Here's how the part is built. I have some questions about the finished solid (model axes, mm). Give positions to 0.01 mm unless a question says otherwise; leave off trailing zeros. Write each loop counter-clockwise with the first axis right and the second up, starting at its lowest first coordinate (ties: lowest second). Pieces come first, ordered by that corner, then holes. Notation, with made-up numbers: (73, 44) - (92, 44) arc R15 ccw to (92, 71) - close; hole circle Ø2 at (77.5, 58). An arc over 180 degrees is marked (long way). Use a Markdown table: item, result.
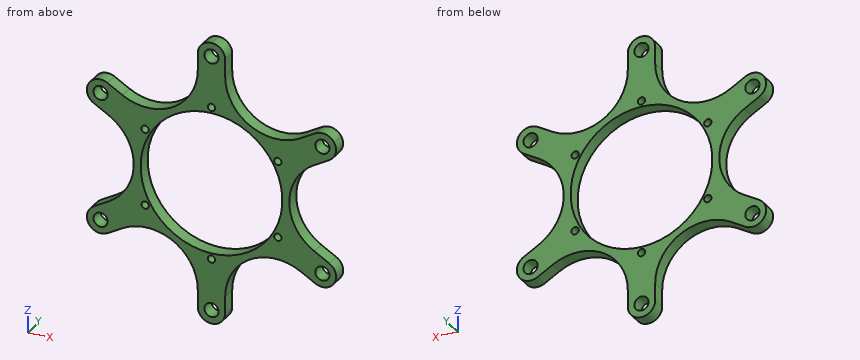
```python
from build123d import *

# Parameters (mm, degrees)
SKETCH_1_R               = 31
EXTRUDE_1_DEPTH          = 6
SKETCH_2_R               = 1.6
SKETCH_2_R_2             = 3.1
CUT_EXTRUDE_1_DEPTH      = 6
PATTERN_CIRCULAR_1_COUNT = 6


with BuildPart() as part:
    # 草图1 → 凸台-拉伸1 (new body)
    with BuildSketch(Plane(origin=(0, 0, 0), x_dir=(1, 0, 0), z_dir=(0, 1, 0))):
        with BuildLine():
            Line((6, 56), (6, 48.497422612))
            ThreePointArc((6, 48.497422612), (17, 29.444863729), (39, 29.444863729))
            Line((39, 29.444863729), (45.497422612, 33.196152423))
            ThreePointArc((45.497422612, 33.196152423), (50.050336883, 33.795554958), (53.693575035, 31))
            ThreePointArc((53.693575035, 31), (54.29297757, 26.447085729), (51.497422612, 22.803847577))
            Line((51.497422612, 22.803847577), (45, 19.052558883))
            ThreePointArc((45, 19.052558883), (34, 0), (45, -19.052558883))
            Line((45, -19.052558883), (51.497422612, -22.803847577))
            ThreePointArc((51.497422612, -22.803847577), (54.29297757, -26.447085729), (53.693575035, -31))
            ThreePointArc((53.693575035, -31), (50.050336883, -33.795554958), (45.497422612, -33.196152423))
            Line((45.497422612, -33.196152423), (39, -29.444863729))
            ThreePointArc((39, -29.444863729), (17, -29.444863729), (6, -48.497422612))
            Line((6, -48.497422612), (6, -56))
            ThreePointArc((6, -56), (4.242640687, -60.242640687), (0, -62))
            ThreePointArc((0, -62), (-4.242640687, -60.242640687), (-6, -56))
            Line((-6, -56), (-6, -48.497422612))
            ThreePointArc((-6, -48.497422612), (-17, -29.444863729), (-39, -29.444863729))
            Line((-39, -29.444863729), (-45.497422612, -33.196152423))
            ThreePointArc((-45.497422612, -33.196152423), (-50.050336883, -33.795554958), (-53.693575035, -31))
            ThreePointArc((-53.693575035, -31), (-54.29297757, -26.447085729), (-51.497422612, -22.803847577))
            Line((-51.497422612, -22.803847577), (-45, -19.052558883))
            ThreePointArc((-45, -19.052558883), (-34, 0), (-45, 19.052558883))
            Line((-45, 19.052558883), (-51.497422612, 22.803847577))
            ThreePointArc((-51.497422612, 22.803847577), (-54.29297757, 26.447085729), (-53.693575035, 31))
            ThreePointArc((-53.693575035, 31), (-50.050336883, 33.795554958), (-45.497422612, 33.196152423))
            Line((-45.497422612, 33.196152423), (-39, 29.444863729))
            ThreePointArc((-39, 29.444863729), (-17, 29.444863729), (-6, 48.497422612))
            Line((-6, 48.497422612), (-6, 56))
            ThreePointArc((-6, 56), (-4.242640687, 60.242640687), (0, 62))
            ThreePointArc((0, 62), (4.242640687, 60.242640687), (6, 56))
        make_face()
        with Locations(Location((0, 0, 0), (0, 0, 270))):
            Circle(SKETCH_1_R, mode=Mode.SUBTRACT)
    extrude(amount=EXTRUDE_1_DEPTH)

    # 草图2 → 切除-拉伸1 (cut)
    with BuildSketch(Plane(origin=(0, 6, 0), x_dir=(1, 0, 0), z_dir=(0, 1, 0))):
        with Locations(Location((0, 33.5, 0), (0, 0, 270))):
            Circle(SKETCH_2_R)
        with Locations(Location((0, 56, 0), (0, 0, 270))):
            Circle(SKETCH_2_R_2)
    cut_extrude_1 = extrude(amount=-CUT_EXTRUDE_1_DEPTH, mode=Mode.SUBTRACT)

    # 阵列(圆周)1: 切除-拉伸1 ×6 about axis
    pattern_circular_1_axis = Axis((0, 0, 0), (0, 1, 0))
    for i in range(1, PATTERN_CIRCULAR_1_COUNT):
        add(cut_extrude_1.rotate(pattern_circular_1_axis, i * 360 / PATTERN_CIRCULAR_1_COUNT), mode=Mode.SUBTRACT)


solid = part.part
```
Item 1: Will these pins go through, and if not, where does the flat tip stop? pin 1 Ø1 at (x, y) = (15.5, 4) entering from -Z; pin 2 Ø1 at (x, y) = (38, 4) entering from +Z; pin 3 Ø2 at (x, y) = (31, 4) entering from +Z.
Values:
| item | result |
|---|---|
| pin 1 | stops at z = -30.75 |
| pin 2 | stops at z = 29.16 |
| pin 3 | stops at z = 26.86 |
Item 2: If we section it at C-C, the plane z = 28: Write out the boundary of the cut face in (x, y).
Values:
| item | result |
|---|---|
| outline | (-54.5, 0) - (-51.6, 0) - (-51.6, 6) - (-54.5, 6) - close; (-45.4, 0) - (-35.99, 0) - (-35.99, 6) - (-45.4, 6) - close; (-20.01, 0) - (-13.3, 0) - (-13.3, 6) - (-20.01, 6) - close; (13.3, 0) - (20.01, 0) - (20.01, 6) - (13.3, 6) - close; (35.99, 0) - (45.4, 0) - (45.4, 6) - (35.99, 6) - close; (51.6, 0) - (54.5, 0) - (54.5, 6) - (51.6, 6) - close |
Item 3: I need wall thicknesses on line 1 along X through (y, z) = (1.6, -17); line 2 along X through (y, z) = (1.95, 56); line 3 along Z through (x, y) = (37.5, 2.5). Which ranges of each line are inside material? Lowest first, please. Write a range as [from, to].
Values:
| item | result |
|---|---|
| line 1 | x = [-42.04, -30.59], [-27.43, -25.92], [25.92, 27.43], [30.59, 42.04] |
| line 2 | x = [-6, -3.1], [3.1, 6] |
| line 3 | z = [-28.65, -11.91], [11.91, 28.65] |
Item 4: If we section it at D-D, the plane y = 4.95: Count the separate pieces of the cut face and the enclosed holes in it, plus the area to 3 significant figures.
Values:
| item | result |
|---|---|
| separate pieces | 1 |
| enclosed holes | 13 |
| area | 2,740 mm2 |
Item 5: If we section it at B-B, the plane x = -17.5: Write out the boundary of the cut face in (y, z), plus the area to 3 significant figures.
Values:
| item | result |
|---|---|
| outline | (0, -29.16) - (6, -29.16) - (6, -25.59) - (0, -25.59) - close; (0, 25.59) - (6, 25.59) - (6, 29.16) - (0, 29.16) - close |
| area | 42.9 mm2 |
Item 6: If we section it at A-A, the plane z = 0: Write out the boundary of the cut face in (x, y).
Values:
| item | result |
|---|---|
| outline | (-34, 0) - (-31, 0) - (-31, 6) - (-34, 6) - close; (31, 0) - (34, 0) - (34, 6) - (31, 6) - close |
